from build123d import *

# Parameters (mm, degrees)
F0_W     = 1400
F0_H     = 700
F1_DEPTH = 250
F3_DEPTH = 250.001
F5_DEPTH = 250.001


with BuildPart() as f1:
    # F0 (on Top) → F1 (new body)
    with BuildSketch(Plane.XY):
        with Locations((700, 350)):
            Rectangle(F0_W, F0_H)
    extrude(amount=F1_DEPTH)

    # F2 (on face) → F3 (cut, through all)
    with BuildSketch(Plane.XY.offset(250)):
        with BuildLine():
            Line((200, 300), (200, 0))
            Line((200, 0), (1200, 0))
            Line((1200, 0), (1200, 300))
            ThreePointArc((1200, 300), (700, 500), (200, 300))
        make_face()
    extrude(amount=-F3_DEPTH, mode=Mode.SUBTRACT)

    # F4 (on face) → F5 (cut, through all)
    with BuildSketch(Plane.XY.offset(250)):
        with BuildLine():
            ThreePointArc((0, 379.6693311224), (315.0936031242, 616.1135866481), (700, 700))
            Line((700, 700), (0, 700))
            Line((0, 700), (0, 379.6693311224))
        make_face()
        with BuildLine():
            Line((1400, 700), (700, 700))
            ThreePointArc((700, 700), (1084.9063968758, 616.1135866481), (1400, 379.6693311224))
            Line((1400, 379.6693311224), (1400, 700))
        make_face()
    extrude(amount=-F5_DEPTH, mode=Mode.SUBTRACT)


solid = f1.part
Model file for the job. Use its own axes, mm. Give positions to 0.01 mm unless a question says otherwise; leave off trailing zeros. Order: outer loops, then holes, each group sorted by start corner. A loop starts at its lowest first (then second) coordinate and runs counter-clockwise, first axis right, second up. Notation, with made-up numbers: (82.5, -34) - (130.5, -34) arc R21 ccw to (130.5, -2) - close; hole circle Ø8 at (14, -29). An arc over 180 degrees is marked (long way). Return JSON: item names as keys, results as strings.
1) Pull direction X, two halves, no side cores. Call faces 1 (the flat face through (200, 152, 127)), 2 (the flat face through (690, 510, 250)), 3 (the flat face through (1200, 148, 127)), 4 (the flat face through (0, 187, 123)): pulls with the +X half, pulls with the -X half, needs draft (parallel to the pull), parting line crosses it, or undercut.
Geometry says:
{"face 1": "undercut", "face 2": "needs draft", "face 3": "undercut", "face 4": "pulls with the -X half"}
2) Probe line 1 (X direction, y = 57, z = 132); line 2 (X direction, y = 392.5, z = 167.5); line 3 (X direction, y = 615, z = 64.5). List the from-to ranges inside material, lowest first. Write a range as from..to.
Geometry says:
{"line 1": "0..200, 1200..1400", "line 2": "11.29..320.11, 1079.89..1388.71", "line 3": "312.67..1087.33"}
3) Cut at B-B, the plane z = 112. Give the cut face in (x, y), plus the area to 3 significant figures.
Geometry says:
{"outline": "(0, 0) - (200, 0) - (200, 300) arc R725 cw to (1200, 300) - (1200, 0) - (1400, 0) - (1400, 379.67) arc R925 ccw to (0, 379.67) - close", "area": "405,000 mm²"}
4) Cut at C-C, the plane y = 457.5. Give the cut face in (x, z).
Geometry says:
{"outline": "(75.65, 0) - (455.42, 0) - (455.42, 250) - (75.65, 250) - close; (944.58, 0) - (1324.35, 0) - (1324.35, 250) - (944.58, 250) - close"}
5) Cut at A-A, the plane y = 162.5. Give the cut face in (x, z).
Geometry says:
{"outline": "(0, 0) - (200, 0) - (200, 250) - (0, 250) - close; (1200, 0) - (1400, 0) - (1400, 250) - (1200, 250) - close"}
6) Flat gauge pins, fed straight in: P1, Ø12, axis at y = 176, z = 150, coming from the -X side; P2, Ø1, axis at x = 592, z = 91.5, coming from the +Y side; P3, Ø4, axis at x = 617, z = 36, coming from the +Y side; P4, Ø8, axis at x = 1225, z = 56.5, coming from the +Y side. Where does each tip first touch, or does it go through?
Geometry says:
{"P1": "x = 0", "P2": "y = 693.73", "P3": "y = 696.45", "P4": "y = 539.32"}
7) Cut at D-D, the plane x = 1061. Give the cut face in (y, z).
Geometry says:
{"outline": "(403.73, 0) - (626.65, 0) - (626.65, 250) - (403.73, 250) - close"}
